Source: CAD feature listing. Evaluate the final solid. Frame: model axes, mm. A direction names the side the tool comes from. Round coordinates to 2 decimals unless told otherwise and drop trailing zeros. Order: outer loops, then holes, each group sorted by start corner. A loop starts at its lowest first (then second) coordinate and runs counter-clockwise, first axis right, second up. Notation, with made-up numbers: M -32,48.25 L -9,48.25 A5 ccw -9,57.25 Z; hole C 37.5,81 d1. An arc over 180 degrees is marked long. Answer as CSV lines item,"result". Start each with the question number.
Item 1: Line query: line 1 (Z direction, x = -35, y = 25.4); line 2 (Z direction, x = 0, y = 8.5); line 3 (Z direction, x = -45, y = 3). Output: solid intervals per line, ascending. Write a range as [from, to].
Item 2: Section query D-D on y = 12. Return the cut outline in (x, z).
Item 3: Section query B-B on y = 25.5. Return the cut outline in (x, z), plus the area to 3 significant figures.
Item 4: Set-up query: faces 1 (the face through (-32.819, 12.106, -56.685)), 2 (the face through (-36, 22.5, 59)), 3 (the face through (25, 5, -25)), 4 (the face through (-11, 0, 1)). Return all of +Z, -Z, +X, -X, +Y, -Y with unobstructed straight access to the full face (end or side cutting, diameter ignored); none if empty.
Item 5: Section query A-A on z = 0. Return the cut outline in (x, y), plus the area to 3 significant figures.
Item 6: First-contact query: P1, Ø12, axis at y = 5, z = 31, coming from the +X side; P2, Ø2, axis at x = 62.5, y = 9.5, coming from the -Z side; P3, Ø2, axis at y = 20.5, z = 49, coming from the -X side. Flat tips, straight axial feed; report the tip coordinate or a pass-through.
Item 7: Pull-direction query (Z, two-part tool) for faces 5 (the face through (-30.19, 18.83, 52.43)), 6 (the face through (72, 22.5, 0)), 7 (the face through (76.105, 25.035, 0.138)), 8 (the face through (-32.681, 12.106, 56.765)); classes: +Z half, -Z half, draft (parallel to the pull), parting line (faces both ways), or undercut.
Item 8: Section query C-C on x = 0. Return the cut outline in (y, z), plus the area to 3 significant figures.
Autodesk Inventor part; units mm, degrees
ref_plane "YZ Plane" through (0, 0, 0) normal (1, 0, 0) x (0, 1, 0)
ref_plane "XZ Plane" through (0, 0, 0) normal (0, 1, 0) x (-1, 0, 0)
ref_plane "XY Plane" through (0, 0, 0) normal (0, 0, 1) x (1, 0, 0)
sketch "Sketch1" plane through (0, 0, 0) normal (0, 1, 0) x (-1, 0, 0)
  line L0 (0, 0) -> (48.2963, -12.941)
  line L1 (0, 0) -> (50, 0) construction
  line L2 (0, 0) -> (48.2963, 12.941)
  line L3 (0, 0) -> (50, 0) construction
  arc A0 (48.2963, -12.941) -> (48.2963, 12.941) centre (0, 0) ccw
  arc A1 (-12.941, 48.2963) -> (-35.3553, 35.3553) centre (0, 0) ccw
  line L4 (0, 0) -> (-12.941, 48.2963)
  line L5 (0, 0) -> (-35.3553, 35.3553)
  arc A2 (-35.3553, -35.3553) -> (-12.941, -48.2963) centre (0, 0) ccw
  line L6 (0, 0) -> (-35.3553, -35.3553)
  line L7 (0, 0) -> (-12.941, -48.2963)
  circle A3 centre (0, 0) radius 5
  circle A4 centre (0, 0) radius 20
  line L8 (0, 0) -> (34.7014, -49.5587)
  line L9 (0, 0) -> (60.5, 0) construction
  line L10 (0, 0) -> (25.5684, -54.8316)
  line L11 (0, 0) -> (60.5, 0) construction
  line L12 (25.5684, -54.8316) -> (27.6815, -59.3632)
  line L13 (34.7014, -49.5587) -> (37.5693, -53.6545)
  arc A5 (27.6815, -59.3632) -> (37.5693, -53.6545) centre (0, 0) ccw
  circle A6 centre (0, 0) radius 50
  circle A7 centre (0, 0) radius 60
  line L14 (0, 0) -> (25.5684, 54.8316)
  line L15 (25.5684, 54.8316) -> (27.6815, 59.3632)
  arc A8 (37.5693, 53.6545) -> (27.6815, 59.3632) centre (0, 0) ccw
  line L16 (0, 0) -> (34.7014, 49.5587)
  line L17 (34.7014, 49.5587) -> (37.5693, 53.6545)
  line L18 (0, 0) -> (-60.2698, -5.2729)
  line L19 (-60.2698, -5.2729) -> (-65.2508, -5.7087)
  arc A9 (-65.2508, 5.7087) -> (-65.2508, -5.7087) centre (0, 0) ccw
  line L20 (0, 0) -> (-60.2698, 5.2729)
  line L21 (-60.2698, 5.2729) -> (-65.2508, 5.7087)
  point P0 (19.3185, -5.1764)
  point P1 (19.3185, 5.1764)
  point P2 (-5.1764, 19.3185)
  point P3 (-14.1421, 14.1421)
  point P4 (-14.1421, -14.1421)
  point P5 (-5.1764, -19.3185)
  point P6 (8.4524, -18.1262)
  point P7 (11.4715, -16.383)
  point P8 (-35.3553, -35.3553)
  point P9 (-35.3553, 35.3553)
  point P10 (-12.941, 48.2963)
  point P11 (-12.941, -48.2963)
  point P12 (25.3571, -54.3785)
  point P13 (34.4146, -49.1491)
  point P14 (34.4146, 49.1491)
  point P15 (25.3571, 54.3785)
  point P16 (-59.7717, 5.2293)
  point P17 (-59.7717, -5.2293)
  dimension "d0" = 50
  dimension "d1" = 15
  dimension "d2" = 50
  dimension "d3" = 15
  dimension "d4" = 50
  dimension "d7" = 360
  dimension "d9" = 10
  dimension "d10" = 40
  dimension "d11" = 60.5
  dimension "d12" = 55
  dimension "d13" = 60.5
  dimension "d14" = 65
  dimension "d16" = 5
  dimension "d17" = 5
  dimension "d18" = 65.5
  dimension "d25" = 100
  dimension "d26" = 120
  dimension "d29" = 360
extrude "Extrusion2" add sketch "Sketch1" along normal blind 10.4 contours A3 L2 A4 L0 | L0 A4 L8 A3 | A3 L16 A4 L2 | A3 L5 A4 L4 | L4 A4 L14 A3 | A3 L20 A4 L5 | A3 L7 A4 L6 | L6 A4 L18 A3 | A3 L10 A4 L7 | L8 A4 L10 A3 | L14 A4 L16 A3 | L18 A4 L20 A3 | A4 L2 A0 L0 | A4 L5 A1 L4 | A4 L7 A2 L6 | A0 A6 L16 A7 L8 | A1 A6 L20 A7 L14 | A2 A6 L10 A7 L18 | L8 A7 L10 A6 | L14 A7 L16 A6 | L18 A7 L20 A6 | L8 L13 A5 L12 L10 A7 | L14 L15 A8 L17 L16 A7 | L18 L19 A9 L21 L20 A7
sketch "Sketch3" plane through (0, 10.4, 0) normal (0, 1, 0) x (1, 0, 0)
  circle A0 centre (0, 0) radius 5
  arc A1 (65.2508, -5.7087) -> (65.2508, 5.7087) centre (0, 0) ccw
  arc A2 (65.2508, -5.7087) -> (65.2508, 5.7087) centre (0, 0) ccw
  line L0 (65.2508, 5.7087) -> (60.2698, 5.2729)
  line L1 (65.2508, 5.7087) -> (59.7717, 5.2293)
  line L2 (65.2508, -5.7087) -> (60.2698, -5.2729)
  line L3 (59.7717, -5.2293) -> (65.2508, -5.7087)
  arc A3 (60.2698, -5.2729) -> (60.2698, 5.2729) centre (0, 0) ccw
  arc A4 (-27.6815, 59.3632) -> (-37.5693, 53.6545) centre (0, 0) ccw
  line L4 (-37.5693, 53.6545) -> (-34.7014, 49.5587)
  arc A5 (-25.5684, 54.8316) -> (-34.7014, 49.5587) centre (0, 0) ccw
  line L5 (-27.6815, 59.3632) -> (-25.5684, 54.8316)
  arc A6 (-37.5693, -53.6545) -> (-27.6815, -59.3632) centre (0, 0) ccw
  line L6 (-27.6815, -59.3632) -> (-25.5684, -54.8316)
  arc A7 (-34.7014, -49.5587) -> (-25.5684, -54.8316) centre (0, 0) ccw
  line L7 (-37.5693, -53.6545) -> (-34.7014, -49.5587)
  dimension "d40" = 5
  dimension "d41" = 5
  dimension "d42" = 60.5
  dimension "d45" = 360
extrude "Extrusion3" add sketch "Sketch3" along normal blind 17.1 contours L2 A3 L0 A1 | L5 A5 L4 A4 | L7 A7 L6 A6
sketch "Sketch4" plane through (0, 27.5, 0) normal (0, 1, 0) x (1, 0, 0)
  arc A0 (-27.6815, 59.3632) -> (-37.5693, 53.6545) centre (0, 0) ccw
  arc A1 (-27.6815, 59.3632) -> (-37.5693, 53.6545) centre (0, 0) ccw
  line L0 (-27.6815, 59.3632) -> (-29.5833, 63.4415)
  line L1 (-27.6815, 59.3632) -> (-23.1815, 59.3632) construction
  line L2 (-37.5693, 53.6545) -> (-40.1504, 57.3406)
  line L3 (-37.5693, 53.6545) -> (-33.0693, 53.6545) construction
  circle A2 centre (-35, 60.6218) radius 1.75
  arc A3 (-29.5833, 63.4415) -> (-40.1504, 57.3406) centre (-35, 60.6218) ccw
  arc A4 (-40.1504, -57.3406) -> (-29.5833, -63.4415) centre (-35, -60.6218) ccw
  circle A5 centre (-35, -60.6218) radius 1.75
  line L4 (-37.5693, -53.6545) -> (-40.1504, -57.3406)
  line L5 (-27.6815, -59.3632) -> (-29.5833, -63.4415)
  arc A6 (-37.5693, -53.6545) -> (-27.6815, -59.3632) centre (0, 0) ccw
  arc A7 (69.7336, -6.1009) -> (69.7336, 6.1009) centre (70, 0) ccw
  circle A8 centre (70, 0) radius 1.75
  line L6 (65.2508, -5.7087) -> (69.7336, -6.1009)
  line L7 (65.2508, 5.7087) -> (69.7336, 6.1009)
  arc A9 (65.2508, -5.7087) -> (65.2508, 5.7087) centre (0, 0) ccw
  point P0 (0, 0)
  dimension "d50" = 4.5
  dimension "d51" = 115
  dimension "d52" = 4.5
  dimension "d53" = 125
  dimension "d63" = 3.5
  dimension "d66" = 360
  dimension "d70" = 70
extrude "Extrusion5" add sketch "Sketch4" against normal blind 5
sketch "Sketch5" plane through (0, 10.4, 0) normal (0, 1, 0) x (1, 0, 0)
  circle A0 centre (0, 0) radius 14.1
  dimension "d71" = 28.2
extrude "Extrusion6" cut sketch "Sketch5" against normal blind 8.5
fillet "Fillet1" radius 2 3 edges at (-32.75, 0, -56.7247) (-32.75, 0, 56.7247) (65.5, 0, 0)
properties part number "MechSwitch_DielecTopV2"
Results:
1,line 1,"[-66.73, -62.37], [-58.87, -49.99], [49.99, 58.87], [62.37, 66.73]"
1,line 2,"[-60, -50], [-20, -14.1], [14.1, 20], [50, 60]"
1,line 3,"[-39.69, -21.79], [-12.06, 12.06], [21.79, 39.69]"
2,outline,"M -37.57,-53.65 A65.5 ccw -27.68,-59.36 L -25.57,-54.83 A60.5 cw -34.7,-49.56 Z; M -37.57,53.65 L -34.7,49.56 A60.5 cw -25.57,54.83 L -27.68,59.36 A65.5 ccw Z; M 60.27,-5.27 L 65.25,-5.71 A65.5 ccw 65.25,5.71 L 60.27,5.27 A60.5 cw Z"
3,outline,"M -40.15,-57.34 A6.11 ccw long -29.58,-63.44 L -27.68,-59.36 L -25.57,-54.83 A60.5 cw -34.7,-49.56 L -37.57,-53.65 Z; M -40.15,57.34 L -37.57,53.65 L -34.7,49.56 A60.5 cw -25.57,54.83 L -27.68,59.36 L -29.58,63.44 A6.11 ccw long Z; M 60.27,-5.27 L 65.25,-5.71 L 69.73,-6.1 A6.11 ccw long 69.73,6.1 L 65.25,5.71 L 60.27,5.27 A60.5 cw Z; hole C -35,-60.62 d3.5; hole C -35,60.62 d3.5; hole C 70,0 d3.5"
3,area,"475 mm^2"
4,face 1,"-Z, -X, -Y"
4,face 2,"+Z, -X, -Y"
4,face 3,"+Y, -Y"
4,face 4,"+Z, -Z, +X, -X, -Y"
5,outline,"M -60,0 L -5,0 L -5,1.9 L -14.1,1.9 L -14.1,10.4 L -60,10.4 Z; M 5,0 L 20,0 L 20,10.4 L 14.1,10.4 L 14.1,1.9 L 5,1.9 Z; M 50,0 L 63.5,0 A2 ccw 65.5,2 L 65.5,22.5 L 68.25,22.5 L 68.25,27.5 L 60.5,27.5 L 60.5,10.4 L 50,10.4 Z; M 71.75,22.5 L 76.11,22.5 L 76.11,27.5 L 71.75,27.5 Z"
5,area,"855 mm^2"
6,P1,"x = 54.54"
6,P2,"z = -5.56"
6,P3,"x = -35.01"
7,face 5,"undercut"
7,face 6,"draft"
7,face 7,"parting line"
7,face 8,"+Z half"
8,outline,"M 0,-60 L 10.4,-60 L 10.4,-50 L 0,-50 Z; M 0,-20 L 10.4,-20 L 10.4,-14.1 L 1.9,-14.1 L 1.9,-5 L 0,-5 Z; M 0,5 L 1.9,5 L 1.9,14.1 L 10.4,14.1 L 10.4,20 L 0,20 Z; M 0,50 L 10.4,50 L 10.4,60 L 0,60 Z"
8,area,"365 mm^2"
